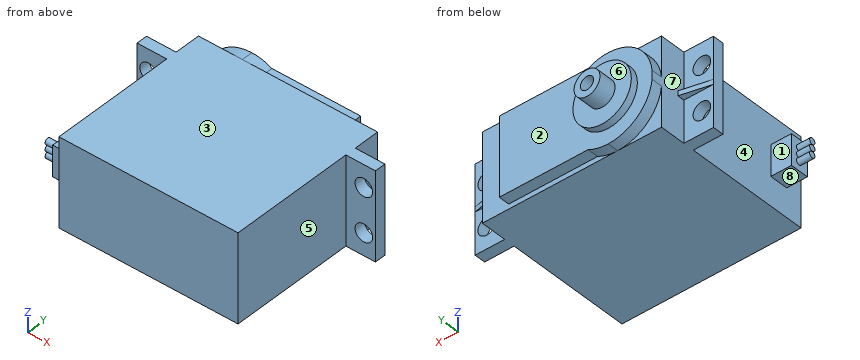
```python
from build123d import *

# Parameters (mm, degrees)
ESQUISSE1_W                       = 40.8
ESQUISSE1_H                       = 39.4
ESQUISSE1_W_2                     = 6.75
ESQUISSE1_H_2                     = 2.5
BOSS_EXTRU_1_DEPTH                = 10.05
DIAM_TRE_DU_PER_AGE_4_0_4_1_D     = 4
BOSS_EXTRU_3_DEPTH                = 0.55
ESQUISSE6_R                       = 6.65
BOSS_EXTRU_4_DEPTH                = 1.6
ESQUISSE4_R                       = 2.95
BOSS_EXTRU_2_DEPTH                = 4
DIAM_TRE_DU_PER_AGE_3_0_3_1_D     = 3
DIAM_TRE_DU_PER_AGE_3_0_3_1_DEPTH = 6
DIAM_TRE_DU_PER_AGE_3_0_3_1_TIP   = 0.901290929
ENL_V_MAT_EXTRU_1_DEPTH           = 2.5
ESQUISSE8_W                       = 7
ESQUISSE8_H                       = 4.2
BOSS_EXTRU_5_DEPTH                = 4.7
ESQUISSE9_R                       = 0.7
BOSS_EXTRU_6_DEPTH                = 3


with BuildPart() as part:
    # Esquisse1 → Boss.-Extru.1 (new, symmetric)
    with BuildSketch(Plane.XY):
        with Locations((0, -8.8)):
            Rectangle(ESQUISSE1_W, ESQUISSE1_H)
        with Locations((-23.775, 1.25)):
            Rectangle(ESQUISSE1_W_2, ESQUISSE1_H_2)
        with Locations((23.775, 1.25)):
            Rectangle(ESQUISSE1_W_2, ESQUISSE1_H_2)
    extrude(amount=BOSS_EXTRU_1_DEPTH, both=True)

    # Diamètre du perçage Ø4.0 (4)1 (through all)
    with Locations(Plane(origin=(0, 2.5, 0), x_dir=(1, 0, 0), z_dir=(0, 1, 0))):
        with Locations((-24.5, 5), (24.5, 5), (24.5, -5), (-24.5, -5)):
            Hole(DIAM_TRE_DU_PER_AGE_4_0_4_1_D / 2)

    # Esquisse5 → Boss.-Extru.3 (add, symmetric)
    with BuildSketch(Plane.XY):
        Polygon((-20.4, 4.1), (-27.15, 2.5), (-20.4, 2.5), align=None)
        Polygon((20.4, 2.5), (20.4, 4.1), (27.15, 2.5), align=None)
    extrude(amount=BOSS_EXTRU_3_DEPTH, both=True)

    # Esquisse6 → Boss.-Extru.4 (add)
    with BuildSketch(Plane(origin=(0, 10.9, 0), x_dir=(1, 0, 0), z_dir=(0, 1, 0))):
        with Locations(Location((-10.4, 0, 0), (0, 0, 180))):
            Circle(ESQUISSE6_R)
    extrude(amount=BOSS_EXTRU_4_DEPTH)

    # Esquisse4 → Boss.-Extru.2 (add)
    with BuildSketch(Plane(origin=(0, 12.5, 0), x_dir=(1, 0, 0), z_dir=(0, 1, 0))):
        with Locations(Location((-10.4, 0, 0), (0, 0, 180))):
            Circle(ESQUISSE4_R)
    extrude(amount=BOSS_EXTRU_2_DEPTH)

    # Diamètre du perçage Ø3.0 (3)1
    with Locations(Plane(origin=(0, 16.5, 0), x_dir=(1, 0, 0), z_dir=(0, 1, 0))):
        with Locations((-10.4, 0)):
            Hole(DIAM_TRE_DU_PER_AGE_3_0_3_1_D / 2, depth=DIAM_TRE_DU_PER_AGE_3_0_3_1_DEPTH)
            with Locations((0, 0, -(DIAM_TRE_DU_PER_AGE_3_0_3_1_DEPTH + DIAM_TRE_DU_PER_AGE_3_0_3_1_TIP / 2))):  # 118° drill point
                Cone(0, DIAM_TRE_DU_PER_AGE_3_0_3_1_D / 2, DIAM_TRE_DU_PER_AGE_3_0_3_1_TIP, mode=Mode.SUBTRACT)

    # Esquisse7 → Enlèv. mat.-Extru.1 (cut)
    with BuildSketch(Plane(origin=(0, 10.9, 0), x_dir=(1, 0, 0), z_dir=(0, 1, 0))):
        with BuildLine():
            ThreePointArc((-20.4, 1.00124922), (-17.143142641, 7.452014984), (-10.4, 10.05))
            Line((-10.4, 10.05), (-20.4, 10.05))
            Line((-20.4, 10.05), (-20.4, 1.00124922))
        make_face()
        with BuildLine():
            Line((-20.4, -10.05), (-10.4, -10.05))
            ThreePointArc((-10.4, -10.05), (-17.143142641, -7.452014984), (-20.4, -1.00124922))
            Line((-20.4, -1.00124922), (-20.4, -10.05))
        make_face()
        with BuildLine():
            ThreePointArc((-10.4, 10.05), (-8.048936411, 9.771130948), (-5.82834822, 8.95))
            Line((-5.82834822, 8.95), (14.4, 8.95))
            Line((14.4, 8.95), (14.4, -8.95))
            Line((14.4, -8.95), (-5.82834822, -8.95))
            ThreePointArc((-5.82834822, -8.95), (-8.048936411, -9.771130948), (-10.4, -10.05))
            Line((-10.4, -10.05), (20.4, -10.05))
            Line((20.4, -10.05), (20.4, 10.05))
            Line((20.4, 10.05), (-10.4, 10.05))
        make_face()
    extrude(amount=-ENL_V_MAT_EXTRU_1_DEPTH, mode=Mode.SUBTRACT)

    # Esquisse8 → Boss.-Extru.5 (add)
    with BuildSketch(Plane.ZY.offset(20.4)):
        with Locations((0, -22.6)):
            Rectangle(ESQUISSE8_W, ESQUISSE8_H)
    extrude(amount=BOSS_EXTRU_5_DEPTH)

    # Esquisse9 → Boss.-Extru.6 (add)
    with BuildSketch(Plane.ZY.offset(25.1)):
        with Locations((-1.5, -22.523764429)):
            Circle(ESQUISSE9_R)
        with Locations((0, -22.523764429)):
            Circle(ESQUISSE9_R)
        with Locations(Location((1.5, -22.523764429, 0), (0, 0, 180))):
            Circle(ESQUISSE9_R)
    extrude(amount=BOSS_EXTRU_6_DEPTH)


solid = part.part
```
Verification items for the finished model (mm, model axes). Face numbers are marked on the shaded views. A direction names the side the tool comes from. Round coordinates to 2 decimals unless told otherwise and drop trailing zeros. Write each loop counter-clockwise with the first axis right and the second up, starting at its lowest first coordinate (ties: lowest second). Pieces come first, ordered by that corner, then holes.
1. Section check C-C on x = 24.5. Enter the section's corners in (y, z), plus the area to 3 significant figures.
2. Section check B-B on z = 5. Enter the section's corners in (x, y), plus the area to 3 significant figures.
3. Section check A-A on y = 1. Enter the section's corners in (x, z).
4. Access from +Z, -Z, +X, -X, +Y, -Y to the whole of each face (thin tool, end or side, straight path). Record for the marked faces 5, 6, 7 and 8.
5. Gauge pin test, flat ends, axial feed: P1, Ø2.5, axis at x = -24.5, z = -5, coming from the +Y side; P2, Ø1.3, axis at x = -22, y = -23, coming from the -Z side; P3, Ø3, axis at x = 0, y = 10, coming from the -Z side; P4, Ø2, axis at x = 24, z = -4, coming from the +Y side. Record the tip position at first contact, or that the pin passes through.
6. Section check D-D on x = -24.5. Enter the section's corners in (y, z).
7. Scan lines: L1, parallel to Z at x = -24.5, y = 1; L2, parallel to Z at x = -24, y = 1; L3, parallel to X at y = -11, z = 5.5. Record each from-to range of solid material in increasing order.
8. Draft check along Y on the marked faces 1, 2, 3 and 4. Enter one of: +Y half, -Y half, draft (parallel to the pull), parting line (faces both ways), or undercut.
Answer:
1. outline: (0, -10.05) - (2.5, -10.05) - (2.5, -7) - (0, -7) - close; (0, -3) - (2.5, -3) - (2.5, -0.55) - (3.13, -0.55) - (3.13, 0.55) - (2.5, 0.55) - (2.5, 3) - (0, 3) - close; (0, 7) - (2.5, 7) - (2.5, 10.05) - (0, 10.05) - close
1. area: 30.9 mm2
2. outline: (-27.15, 0) - (-26.5, 0) - (-26.5, 2.5) - (-27.15, 2.5) - close; (-22.5, 0) - (-20.4, 0) - (-20.4, -28.5) - (20.4, -28.5) - (20.4, 0) - (22.5, 0) - (22.5, 2.5) - (20.4, 2.5) - (20.4, 8.4) - (14.4, 8.4) - (14.4, 10.9) - (-6.02, 10.9) - (-6.02, 12.5) - (-14.78, 12.5) - (-14.78, 10.9) - (-19.12, 10.9) - (-19.12, 8.4) - (-20.4, 8.4) - (-20.4, 2.5) - (-22.5, 2.5) - close; (26.5, 0) - (27.15, 0) - (27.15, 2.5) - (26.5, 2.5) - close
2. area: 1,620 mm2
3. outline: (-27.15, -10.05) - (27.15, -10.05) - (27.15, 10.05) - (-27.15, 10.05) - close; hole circle Ø4 at (-24.5, -5); hole circle Ø4 at (-24.5, 5); hole circle Ø4 at (24.5, -5); hole circle Ø4 at (24.5, 5)
4. face 5: +Z, -Z, +X, -Y
4. face 6: +Y
4. face 7: -X, +Y
4. face 8: -Z, -X, -Y
5. P1: passes through
5. P2: stops at z = -3.5
5. P3: stops at z = -8.95
5. P4: stops at y = 2.5
6. outline: (-24.7, -3.5) - (-20.5, -3.5) - (-20.5, 3.5) - (-24.7, 3.5) - close; (0, -10.05) - (2.5, -10.05) - (2.5, -7) - (0, -7) - close; (0, -3) - (2.5, -3) - (2.5, -0.55) - (3.13, -0.55) - (3.13, 0.55) - (2.5, 0.55) - (2.5, 3) - (0, 3) - close; (0, 7) - (2.5, 7) - (2.5, 10.05) - (0, 10.05) - close
7. L1: z = -10.05 to -7, -3 to 3, 7 to 10.05
7. L2: z = -10.05 to -6.94, -3.06 to 3.06, 6.94 to 10.05
7. L3: x = -20.4 to 20.4
8. face 1: undercut
8. face 2: +Y half
8. face 3: draft
8. face 4: undercut
